For this review, take the finished solid that the model builds, in its own axes (mm). A direction names the side the tool comes from. Round coordinates to 2 decimals unless told otherwise and drop trailing zeros. Write each loop counter-clockwise with the first axis right and the second up, starting at its lowest first coordinate (ties: lowest second). Pieces come first, ordered by that corner, then holes. Notation, with made-up numbers: (-37.75, -28) -> (13.25, -28) arc R31 cw to (13.25, -4) -> close; hole circle Ø1 at (-13, 74). An arc over 180 degrees is marked (long way). Write item = value, one per line. Start each with the question number.
```python
from build123d import *

# Parameters (mm, degrees)
F0_W      = 50
F0_H      = 50
F1_DEPTH  = 3.5
F2_W      = 3.5
F2_H      = 20
F3_DEPTH  = 25
F5_DEPTH  = 25
F6_R      = 5.9215
F7_DEPTH  = 1.6
F8_R      = 3.0875
F9_DEPTH  = 25
F10_R     = 5.9215
F11_DEPTH = 1.6


with BuildPart() as f1:
    # F0 (on Front) → F1 (new body)
    with BuildSketch(Plane.XZ):
        Rectangle(F0_W, F0_H)
    extrude(amount=F1_DEPTH)

    # F2 (on Top) → F3 (join, symmetric)
    with BuildSketch(Plane.XY):
        with Locations((-4.25, 10)):
            Rectangle(F2_W, F2_H)
    extrude(amount=F3_DEPTH, both=True)

    # F4 (on face) → F5 (cut)
    with BuildSketch(Plane(origin=(-6, 0, 0), x_dir=(0, -1, 0), z_dir=(-1, 0, 0))):
        with BuildLine():
            Line((-10, 7.5), (-6.9125, 7.5))
            ThreePointArc((-6.9125, 7.5), (-12.183192, 9.683192), (-10, 4.4125))
            Line((-10, 4.4125), (-10, 7.5))
        make_face()
        with BuildLine():
            ThreePointArc((-6.9125, -7.5), (-7.816808, -5.316808), (-10, -4.4125))
            Line((-10, -4.4125), (-10, -7.5))
            Line((-10, -7.5), (-6.9125, -7.5))
        make_face()
        with BuildLine():
            Line((-10, -7.5), (-10, -4.4125))
            ThreePointArc((-10, -4.4125), (-12.183192, -9.683192), (-6.9125, -7.5))
            Line((-6.9125, -7.5), (-10, -7.5))
        make_face()
        with BuildLine():
            ThreePointArc((-10, 4.4125), (-7.816808, 5.316808), (-6.9125, 7.5))
            Line((-6.9125, 7.5), (-10, 7.5))
            Line((-10, 7.5), (-10, 4.4125))
        make_face()
    extrude(amount=-F5_DEPTH, mode=Mode.SUBTRACT)

    # F6 (on face) → F7 (cut)
    with BuildSketch(Plane(origin=(-6, 0, 0), x_dir=(0, -1, 0), z_dir=(-1, 0, 0))):
        with Locations((-10, 7.5)):
            Circle(F6_R)
        with Locations((-10, -7.5)):
            Circle(F6_R)
    extrude(amount=-F7_DEPTH, mode=Mode.SUBTRACT)

    # F8 (on face) → F9 (cut)
    with BuildSketch(Plane(origin=(0, 0, 0), x_dir=(-1, 0, 0), z_dir=(0, 1, 0))):
        with Locations((-15, 7.5)):
            Circle(F8_R)
        with Locations((-15, -7.5)):
            Circle(F8_R)
        with Locations((15, 7.5)):
            Circle(F8_R)
        with Locations((15, -7.5)):
            Circle(F8_R)
    extrude(amount=-F9_DEPTH, mode=Mode.SUBTRACT)

    # F10 (on face) → F11 (cut)
    with BuildSketch(Plane(origin=(0, 0, 0), x_dir=(-1, 0, 0), z_dir=(0, 1, 0))):
        with Locations((-15, 7.5)):
            Circle(F10_R)
        with Locations((-15, -7.5)):
            Circle(F10_R)
        with Locations((15.092427, 7.5)):
            Circle(F10_R)
        with Locations((15, -7.5)):
            Circle(F10_R)
    extrude(amount=-F11_DEPTH, mode=Mode.SUBTRACT)


solid = f1.part
```
1. Consider section B-B, the plane z = -20. Give the boundary of the cut face in (x, y), then the cut area to 3 significant figures.
2. Wall thickness on L1, parallel to Z at x = 15, y = -2.1; L2, parallel to Z at x = 15, y = -0.65; L3, parallel to X at y = 2, z = 6: over which ranges is each line inside the solid? List them lowest first. Write a range as from..to.
3. Machinability: for faces 4 (the flat face through (-18, -1.6, -10)), 5 (the flat face through (-16, 0, 0)), 6 (the flat face through (-2.5, 10, 0)), 7 (the flat face through (-4.4, 7, 5)), which of the approach directions +Z, -Z, +X, -X, +Y, -Y give a long, thin tool a straight path to every point of the face, cutting with its end or side? Answer none if there is none.
4. Consider section A-A, the plane x = 15. Give the boundary of the cut face in (y, z), then the cut area to 3 significant figures.
5. Consider section C-C, the plane z = 8.5. Give the number of separate pieces and of enclosed holes in the cut face, then the cut area to 3 significant figures.
6. Draft analysis for pull direction Z (two halves, no side actions). For faces 1 (the flat face through (-25, -2, 0)), 2 (the flat face through (-18, -1.6, 5)), 3 (the flat face through (-2, -0.4, 25)), state which applies: +Z half, -Z half, draft (parallel to the pull), parting line (faces both ways), or undercut.
7. Clearance check with flat-ended pins moving along their axes: pin 1 Ø9.5 at (y, z) = (10, -7.5) entering from +X; pin 2 Ø5 at (y, z) = (8.5, 2.5) entering from -X; pin 3 Ø9.5 at (x, z) = (-14.5, 7.5) entering from +Y; pin 4 Ø1 at (y, z) = (10, 5.5) entering from +X. State where each tip first meets the part, or that it passes through.
Outcome:
q1.outline = (-25, -3.5) -> (25, -3.5) -> (25, 0) -> (-2.5, 0) -> (-2.5, 20) -> (-6, 20) -> (-6, 0) -> (-25, 0) -> close
q1.area = 245 mm2
q2.L1 = -25..-10.59, -4.41..4.41, 10.59..25
q2.L2 = -25..-13.42, -1.58..1.58, 13.42..25
q2.L3 = -6..-2.5
q3.face_4 = +Y
q3.face_5 = +Z, -Z, -X, +Y
q3.face_6 = +Z, -Z, +X, +Y
q3.face_7 = -X
q4.outline = (-3.5, -25) -> (0, -25) -> (0, -13.42) -> (-1.6, -13.42) -> (-1.6, -10.59) -> (-3.5, -10.59) -> close; (-3.5, -4.41) -> (-1.6, -4.41) -> (-1.6, -1.58) -> (0, -1.58) -> (0, 1.58) -> (-1.6, 1.58) -> (-1.6, 4.41) -> (-3.5, 4.41) -> close; (-3.5, 10.59) -> (-1.6, 10.59) -> (-1.6, 13.42) -> (0, 13.42) -> (0, 25) -> (-3.5, 25) -> close
q4.area = 114 mm2
q5.separate_pieces = 4
q5.enclosed_holes = 0
q5.area = 156 mm2
q6.face_1 = draft
q6.face_2 = undercut
q6.face_3 = +Z half
q7.pin_1 = -2.5
q7.pin_2 = -6
q7.pin_3 = -1.6
q7.pin_4 = through
